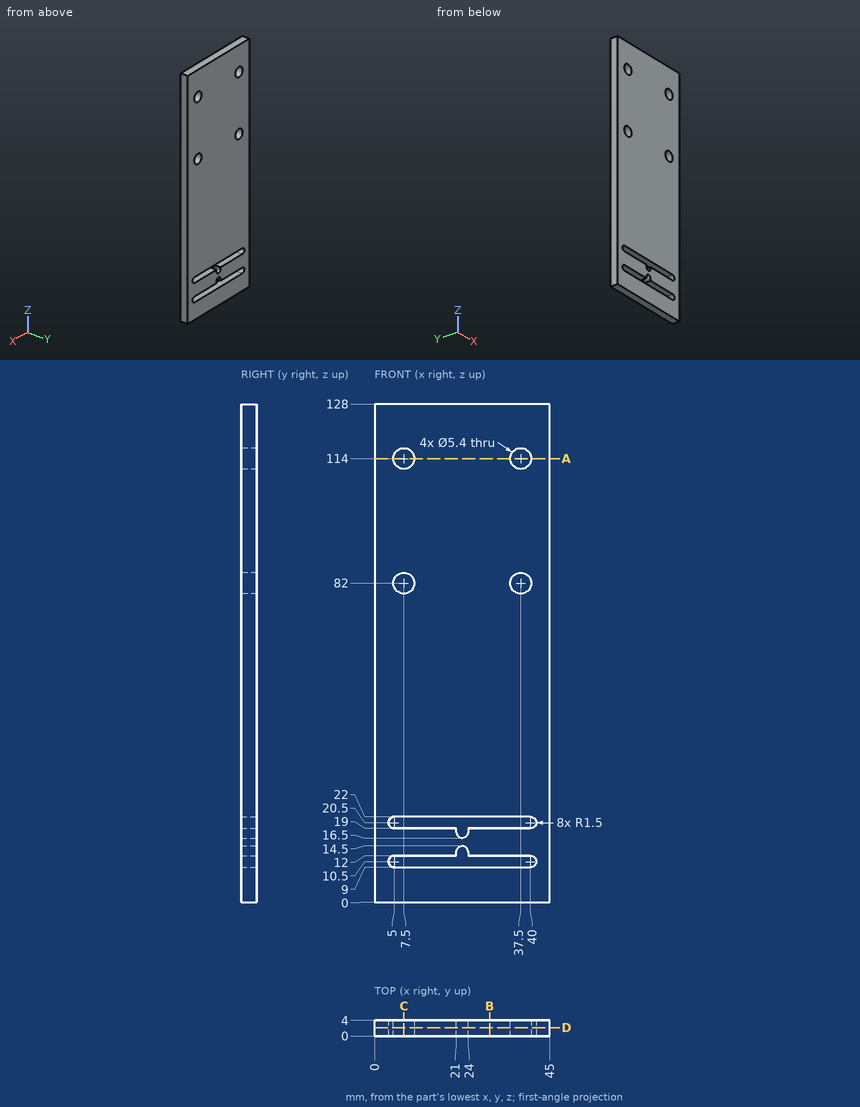
Design review of the part shown in the three views and the two pictorial views. Dimensions are in mm from the part's minimum x, y and z. Round coordinates to 2 decimals unless told otherwise and drop trailing zeros. Write each loop counter-clockwise with the first axis right and the second up, starting at its lowest first coordinate (ties: lowest second). Pieces come first, ordered by that corner, then holes. Notation, with made-up numbers: (-35, 8.5) -> (16, 8.5) arc R29 ccw to (16, 42.5) -> close; hole circle Ø2 at (23.25, 22). An arc over 180 degrees is marked (long way). Write item = value, one per line. Start each with the question number.
1) Take a section at C-C, the plane x = 7.5. State the section outline as (y, z) points, plus the area to 3 significant figures.
2) Take a section at B-B, the plane x = 29.5. State the section outline as (y, z) points, plus the area to 3 significant figures.
3) Clearance check with flat-ended pins moving along their axes: pin 1 (7 mm diameter, centred on x = 37.5, z = 114, fed in from -Y); pin 2 (4.5 mm diameter, centred on x = 37.5, z = 82, fed in from -Y). State where each tip first meets the part, or that it passes through.
4) Wall thickness on probe 1 along Z at (x, y) = (11, 2.3); probe 2 along Z at (x, y) = (7.5, 2.4); probe 3 along Z at (x, y) = (4, 3.05): over which ranges is each line inside the solid? List them lowest first. Write a range as from..to.
5) Take a section at A-A, the plane z = 114. State the section outline as (x, y) points.
6) Take a section at D-D, the plane y = 2.15. Count the separate pieces of the cut face and the enclosed holes in it, plus the area to 3 significant figures.
Results list:
q1.outline = (0, 0) -> (4, 0) -> (4, 9) -> (0, 9) -> close; (0, 12) -> (4, 12) -> (4, 19) -> (0, 19) -> close; (0, 22) -> (4, 22) -> (4, 79.3) -> (0, 79.3) -> close; (0, 84.7) -> (4, 84.7) -> (4, 111.3) -> (0, 111.3) -> close; (0, 116.7) -> (4, 116.7) -> (4, 128) -> (0, 128) -> close
q1.area = 445 mm²
q2.outline = (0, 0) -> (4, 0) -> (4, 9) -> (0, 9) -> close; (0, 12) -> (4, 12) -> (4, 19) -> (0, 19) -> close; (0, 22) -> (4, 22) -> (4, 128) -> (0, 128) -> close
q2.area = 488 mm²
q3.pin_1 = 0
q3.pin_2 = through
q4.probe_1 = 0..9, 12..19, 22..128
q4.probe_2 = 0..9, 12..19, 22..79.3, 84.7..111.3, 116.7..128
q4.probe_3 = 0..9.38, 11.62..19.38, 21.62..128
q5.outline = (0, 0) -> (4.8, 0) -> (4.8, 4) -> (0, 4) -> close; (10.2, 0) -> (34.8, 0) -> (34.8, 4) -> (10.2, 4) -> close; (40.2, 0) -> (45, 0) -> (45, 4) -> (40.2, 4) -> close
q6.separate_pieces = 1
q6.enclosed_holes = 6
q6.area = 5,430 mm²
